```python
from build123d import *

# Parameters (mm, degrees)
SKETCH1_R           = 27.5
SKETCH1_R_2         = 1.5
SKETCH1_R_3         = 7.5
SKETCH1_W           = 10
SKETCH1_H           = 4
BOSS_EXTRUDE1_DEPTH = 1


with BuildPart() as part:
    # Sketch1 → Boss-Extrude1 (new body)
    with BuildSketch(Plane(origin=(0, 0, 0), x_dir=(1, 0, 0), z_dir=(0, 1, 0))):
        with Locations(Location((0, 0, 0), (0, 0, 270))):
            Circle(SKETCH1_R)
        with Locations(Location((0, 12.5, 0), (0, 0, 270))):
            Circle(SKETCH1_R_2, mode=Mode.SUBTRACT)
        with Locations(Location((12.5, 0, 0), (0, 0, 270))):
            Circle(SKETCH1_R_2, mode=Mode.SUBTRACT)
        with Locations(Location((0, -12.5, 0), (0, 0, 270))):
            Circle(SKETCH1_R_2, mode=Mode.SUBTRACT)
        with Locations(Location((-12.5, 0, 0), (0, 0, 270))):
            Circle(SKETCH1_R_2, mode=Mode.SUBTRACT)
        with Locations(Location((0, 0, 0), (0, 0, 270))):
            Circle(SKETCH1_R_3, mode=Mode.SUBTRACT)
        with Locations((0, 23.086362523)):
            Rectangle(SKETCH1_W, SKETCH1_H, mode=Mode.SUBTRACT)
    extrude(amount=BOSS_EXTRUDE1_DEPTH)


solid = part.part
```
Geometry check sheet. Reference: the model listing, model coordinates, mm. Give positions to 0.01 mm unless a question says otherwise; leave off trailing zeros. Write each loop counter-clockwise with the first axis right and the second up, starting at its lowest first coordinate (ties: lowest second). Pieces come first, ordered by that corner, then holes.
1) Section check A-A, the plane z = 0. Record the boundary of the cut face in (x, y), and give its area (3 significant figures).
2) Material ranges on L1, parallel to X at y = 0.5, z = 0; L2, parallel to X at y = 0.6, z = -0.5; L3, parallel to Z at x = -4, y = 0.1, recorded low to high.
3) Gauge pin test, flat end, axial feed: pin 1 (2.5 mm diameter, centred on x = -12.5, z = 0, fed in from -Y). Record the tip position at first contact, or that the pin passes through.
4) Section check C-C, the plane y = 0.3. Record the boundary of the cut face in (x, z), and give its area (3 significant figures).
5) Release check for a two-part mould opening along Z. For faces 1 (the cylindrical face through (-12.05, 0.49, 1.43)), 2 (the flat face through (-6, 1, 6)), 3 (the cylindrical face through (-24.397, 0.493, 12.69)) record: pulls with the +Z half, pulls with the -Z half, needs draft (parallel to the pull), parting line crosses it, or undercut.
6) Section check B-B, the plane x = 0. Record the boundary of the cut face in (y, z), and give its area (3 significant figures).
7) Section check D-D, the plane x = 12.5. Record the boundary of the cut face in (y, z).
Computed:
1. outline: (-27.5, 0) - (-14, 0) - (-14, 1) - (-27.5, 1) - close; (-11, 0) - (-7.5, 0) - (-7.5, 1) - (-11, 1) - close; (7.5, 0) - (11, 0) - (11, 1) - (7.5, 1) - close; (14, 0) - (27.5, 0) - (27.5, 1) - (14, 1) - close
1. area: 34.0 mm2
2. L1: x = -27.5 to -14, -11 to -7.5, 7.5 to 11, 14 to 27.5
2. L2: x = -27.5 to -13.91, -11.09 to -7.48, 7.48 to 11.09, 13.91 to 27.5
2. L3: z = -27.21 to -25.09, -21.09 to -6.34, 6.34 to 27.21
3. pin 1: passes through
4. outline: circle Ø55 at (0, 0); hole circle Ø3 at (-12.5, 0); hole circle Ø15 at (0, 0); hole (-5, -25.09) - (5, -25.09) - (5, -21.09) - (-5, -21.09) - close; hole circle Ø3 at (0, -12.5); hole circle Ø3 at (0, 12.5); hole circle Ø3 at (12.5, 0)
4. area: 2,130 mm2
5. face 1: undercut
5. face 2: needs draft
5. face 3: parting line crosses it
6. outline: (0, -27.5) - (1, -27.5) - (1, -25.09) - (0, -25.09) - close; (0, -21.09) - (1, -21.09) - (1, -14) - (0, -14) - close; (0, -11) - (1, -11) - (1, -7.5) - (0, -7.5) - close; (0, 7.5) - (1, 7.5) - (1, 11) - (0, 11) - close; (0, 14) - (1, 14) - (1, 27.5) - (0, 27.5) - close
6. area: 30.0 mm2
7. outline: (0, -24.49) - (1, -24.49) - (1, -1.5) - (0, -1.5) - close; (0, 1.5) - (1, 1.5) - (1, 24.49) - (0, 24.49) - close
